```python
from build123d import *

# Parameters (mm, degrees)
ESQUISSE2_R             = 1.25
ESQUISSE2_R_2           = 1.5
ENL_V_MAT_EXTRU_1_DEPTH = 8


with BuildPart() as part:
    # Esquisse1 → Révolution1 (revolve)
    with BuildSketch(Plane.XY):
        Polygon((-12.5, 8), (-31, 8), (-31, 3), (-22.5, 3), (-22.5, 0), (-12.5, 0), (-12.5, 7.91388756), align=None)
    revolve(axis=Axis((0, 10, 0), (0, -1, 0)))

    # Esquisse2 → Enlèv. mat.-Extru.1 (cut)
    with BuildSketch(Plane(origin=(0, 8, 0), x_dir=(1, 0, 0), z_dir=(0, 1, 0))):
        with Locations(Location((-16, 22, 0), (0, 0, 180))):
            Circle(ESQUISSE2_R)
        with Locations(Location((16, 22, 0), (0, 0, 180))):
            Circle(ESQUISSE2_R)
        with Locations(Location((16, -22, 0), (0, 0, 180))):
            Circle(ESQUISSE2_R)
        with Locations(Location((-16, -22, 0), (0, 0, 180))):
            Circle(ESQUISSE2_R)
        with Locations(Location((-8, 15, 0), (0, 0, 180))):
            Circle(ESQUISSE2_R_2)
        with Locations(Location((8, -15, 0), (0, 0, 180))):
            Circle(ESQUISSE2_R_2)
    extrude(amount=-ENL_V_MAT_EXTRU_1_DEPTH, mode=Mode.SUBTRACT)


solid = part.part
```
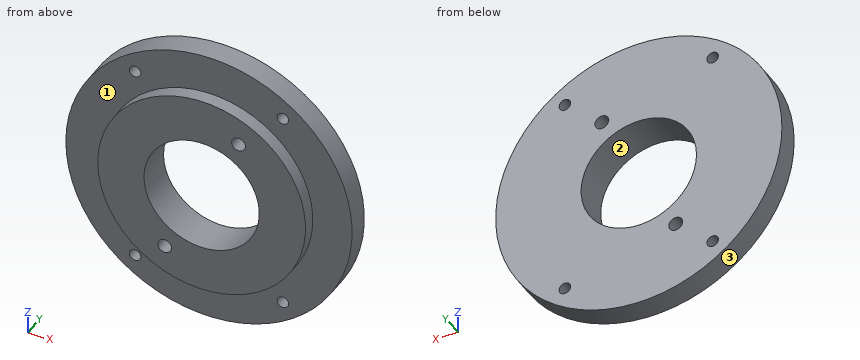
Part model, mm, in its own coordinate system. Face numbers are marked on the shaded views. Round coordinates to 2 decimals unless told otherwise and drop trailing zeros. Order: outer loops, then holes, each group sorted by start corner. A loop starts at its lowest first (then second) coordinate and runs counter-clockwise, first axis right, second up. Notation, with made-up numbers: M -27,2 L 5,2 A27 cw 5,38 Z; hole C 78,-27 d5. An arc over 180 degrees is marked long. Answer in a Markdown table with one row per item. Add a question column.
Q1. Cut at C-C on y = 6. Give the cut face in (x, z), and give its area (3 significant figures).
Q2. Pin check, flat tips, straight feed: pin 1 (1 mm diameter, centred on y = 4, z = -15, fed in from -X); pin 2 (2 mm diameter, centred on x = -16, z = -22, fed in from -Y); pin 3 (3 mm diameter, centred on x = -16, z = 22, fed in from +Y); pin 4 (1 mm diameter, centred on x = -9, y = 4.5, fed in from -Z). Stop position of each tip, or through.
Q3. Cut at D-D on x = 8. Give the cut face in (y, z), and give its area (3 significant figures).
Q4. Wall check: L1, parallel to Z at x = 16, y = 6.35; L2, parallel to Z at x = 0, y = 3.25; L3, parallel to Z at x = -8, y = 5.25. Give the ranges that are in metal, low to high. Write a range as from..to.
Q5. Cut at A-A on x = 0. Give the cut face in (y, z), and give its area (3 significant figures).
Q6. Cut at B-B on z = 0. Give the cut face in (x, y), and give its area (3 significant figures).
Q7. Mould opens along X. For the marked faces 1, 2 and 3 say: +X half, -X half, draft (parallel to the pull), parting line (faces both ways), or undercut.
Established:
| question | item | result |
|---|---|---|
| 1 | outline | C 0,0 d62; hole C -16,-22 d2.5; hole C -16,22 d2.5; hole C 0,0 d25; hole C -8,-15 d3; hole C 8,15 d3; hole C 16,-22 d2.5; hole C 16,22 d2.5 |
| 1 | area | 2,490 mm2 |
| 2 | pin 1 | stops at x = -27.4 |
| 2 | pin 2 | passes through |
| 2 | pin 3 | stops at y = 8 |
| 2 | pin 4 | stops at z = -29.81 |
| 3 | outline | M 0,-21.03 L 3,-21.03 L 3,-29.95 L 8,-29.95 L 8,-9.6 L 0,-9.6 Z; M 0,9.6 L 8,9.6 L 8,13.5 L 0,13.5 Z; M 0,16.5 L 8,16.5 L 8,29.95 L 3,29.95 L 3,21.03 L 0,21.03 Z |
| 3 | area | 248 mm2 |
| 4 | L1 | z = -26.55..-23.25, -20.75..20.75, 23.25..26.55 |
| 4 | L2 | z = -31..-12.5, 12.5..31 |
| 4 | L3 | z = -29.95..-16.5, -13.5..-9.6, 9.6..29.95 |
| 5 | outline | M 0,-22.5 L 3,-22.5 L 3,-31 L 8,-31 L 8,-12.5 L 0,-12.5 Z; M 0,12.5 L 8,12.5 L 8,31 L 3,31 L 3,22.5 L 0,22.5 Z |
| 5 | area | 245 mm2 |
| 6 | outline | M -31,3 L -22.5,3 L -22.5,0 L -12.5,0 L -12.5,8 L -31,8 Z; M 12.5,0 L 22.5,0 L 22.5,3 L 31,3 L 31,8 L 12.5,8 Z |
| 6 | area | 245 mm2 |
| 7 | face 1 | draft |
| 7 | face 2 | undercut |
| 7 | face 3 | parting line |
